```python
from build123d import *

# Parameters (mm, degrees)
F0_W      = 80.8736
F0_H      = 50.8
F1_DEPTH  = 37.592
F3_DEPTH  = 31.242
F4_W      = 30.85465
F4_H      = 38.89375
F5_DEPTH  = 31.242
F6_R      = 6.35
F7_DEPTH  = 25400
F8_DEPTH  = 31.242
F9_R      = 1.89865
F10_DEPTH = 25.4
F11_R     = 3.3782
F12_DEPTH = 25.4


# Not quite as in the source:
# - a feature names something its author has since deleted; it is built from what else it names


with BuildPart() as f1:
    # F0 (on Top) → F1 (new body)
    with BuildSketch(Plane.XY):
        Rectangle(F0_W, F0_H)
    extrude(amount=F1_DEPTH)

    # F2 (on face) → F3 (cut)
    with BuildSketch(Plane.XY.offset(37.592)):
        Polygon((40.4368, 25.4), (21.3868, 25.4), (21.3868, 19.05), (21.3868, -19.05), (21.3868, -25.4), (40.4368, -25.4), (40.4368, -19.05), (40.4368, 19.05), align=None)
    extrude(amount=-F3_DEPTH, mode=Mode.SUBTRACT)

    # F4 (on face) → F5 (cut)
    with BuildSketch(Plane(origin=(0, 0, 0), x_dir=(1, 0, 0), z_dir=(0, 0, -1))):
        Rectangle(F4_W, F4_H)
    extrude(amount=-F5_DEPTH, mode=Mode.SUBTRACT)

    # F6 (on face) → F7 (cut)
    with BuildSketch(Plane.XZ.offset(25.4)):
        with Locations((0, 16.51)):
            Circle(F6_R)
    extrude(amount=-F7_DEPTH, mode=Mode.SUBTRACT)

    # F2 (on face) → F8 (cut)
    with BuildSketch(Plane.XY.offset(37.592)):
        Polygon((-40.4368, 25.4), (-40.4368, 19.05), (-40.4368, -19.05), (-40.4368, -25.4), (-21.3868, -25.4), (-21.3868, -19.05), (-21.3868, 19.05), (-21.3868, 25.4), align=None)
    extrude(amount=-F8_DEPTH, mode=Mode.SUBTRACT)

    # F9 (on face) → F10 (cut)
    with BuildSketch(Plane.XY.offset(37.592)):
        with Locations((0, 14.14145)):
            Circle(F9_R)
        with Locations((0, -14.12875)):
            Circle(F9_R)
    extrude(amount=-F10_DEPTH, mode=Mode.SUBTRACT)

    # F11 (on face) → F12 (cut)
    with BuildSketch(Plane.XY.offset(6.35)):
        with Locations((-30.7086, 15.6718)):
            Circle(F11_R)
        with Locations((-30.7086, -15.6718)):
            Circle(F11_R)
        with Locations((30.7086, 15.6718)):
            Circle(F11_R)
        with Locations((30.7086, -15.6718)):
            Circle(F11_R)
    extrude(amount=-F12_DEPTH, mode=Mode.SUBTRACT)


solid = f1.part
```
The listing builds one solid part. Answer for the finished solid, in the listing's coordinates (mm). A direction names the side the tool comes from. Give positions to 0.01 mm unless a question says otherwise; leave off trailing zeros. Order: outer loops, then holes, each group sorted by start corner. A loop starts at its lowest first (then second) coordinate and runs counter-clockwise, first axis right, second up. Notation, with made-up numbers: M 78,-13.5 L 93,-13.5 A25 cw 93,22.5 Z; hole C -40,78.25 d5. An arc over 180 degrees is marked long. Put each result on its own line as item: value. Start each with the question number.
Item 1: For a pull along X with two mould halves and no side action, classify faces 1 (the face through (27.334, 15.82, 3.219)), 2 (the face through (40.437, 0, 3)), 3 (the face through (-31, 0, 6.35)) as +X half, -X half, draft (parallel to the pull), parting line (faces both ways), or undercut.
Item 2: Flat-ended cylindrical pins translate along their axes: P1, Ø8, axis at x = -30.71, y = -15.67, coming from the +Z side; P2, Ø6, axis at y = -7, z = 19, coming from the -X side; P3, Ø15.5, axis at y = 2, z = 27.5, coming from the +X side. Find the tip coordinate at first contact, or state that the pin passes through.
Item 3: Find the intervals of material crossed by line 1 along X through (y, z) = (15.5, 2); line 2 along X through (y, z) = (21, 16); line 3 along X through (y, z) = (16.5, 23), in increasing order.
Item 4: The part is cut by section B-B, the plane x = 0. Determine the outline of the cut face in (y, z).
Item 5: The part is cut by section D-D, the plane z = 25. Determine the outline of the cut face in (x, y), and give its area (3 significant figures).
Item 6: The part is cut by section A-A, the plane z = 16.51. Determine the outline of the cut face in (x, y), and give its area (3 significant figures).
Item 7: Which of the six approach directions +Z, -Z, +X, -X, +Y, -Y give full straight-line access (tool end or side, diameter ignored) to faces 4 (the face through (21.387, 0, 22)), 5 (the face through (0, 0, 31.242)), 6 (the face through (-0.412, 12.288, 34.461))?
Item 8: The part is cut by section C-C, the plane y = 4.5. Determine the outline of the cut face in (x, z), and give its area (3 significant figures).
Answer key:
1. face 1: undercut
1. face 2: +X half
1. face 3: draft
2. P1: stops at z = 6.35
2. P2: stops at x = -21.39
2. P3: stops at x = 21.39
3. line 1: x = -40.44 to -34.08, -27.33 to -15.43, 15.43 to 27.33, 34.08 to 40.44
3. line 2: x = -21.39 to -6.33, 6.33 to 21.39
3. line 3: x = -21.39 to -15.43, 15.43 to 21.39
4. outline: M -25.4,0 L -19.45,0 L -19.45,10.16 L -25.4,10.16 Z; M -25.4,22.86 L -19.45,22.86 L -19.45,31.24 L -16.03,31.24 L -16.03,37.59 L -25.4,37.59 Z; M -12.23,31.24 L 12.24,31.24 L 12.24,37.59 L -12.23,37.59 Z; M 16.04,31.24 L 19.45,31.24 L 19.45,22.86 L 25.4,22.86 L 25.4,37.59 L 16.04,37.59 Z; M 19.45,0 L 25.4,0 L 25.4,10.16 L 19.45,10.16 Z
5. outline: M -21.39,-25.4 L 21.39,-25.4 L 21.39,25.4 L -21.39,25.4 Z; hole M -15.43,-19.45 L 15.43,-19.45 L 15.43,19.45 L -15.43,19.45 Z
5. area: 973 mm²
6. outline: M -21.39,-25.4 L -6.35,-25.4 L -6.35,-19.45 L -15.43,-19.45 L -15.43,19.45 L -6.35,19.45 L -6.35,25.4 L -21.39,25.4 Z; M 6.35,-25.4 L 21.39,-25.4 L 21.39,25.4 L 6.35,25.4 L 6.35,19.45 L 15.43,19.45 L 15.43,-19.45 L 6.35,-19.45 Z
6. area: 822 mm²
7. face 4: +Z, +X, +Y, -Y
7. face 5: -Z
7. face 6: +Z, -Z
8. outline: M -40.44,0 L -15.43,0 L -15.43,31.24 L 15.43,31.24 L 15.43,0 L 40.44,0 L 40.44,6.35 L 21.39,6.35 L 21.39,37.59 L -21.39,37.59 L -21.39,6.35 L -40.44,6.35 Z
8. area: 886 mm²
